```python
from build123d import *

# Parameters (mm, degrees)
SKETCH1_W           = 38
SKETCH1_H           = 26
BOSS_EXTRUDE1_DEPTH = 2
SKETCH4_W           = 29.4
SKETCH4_H           = 21.4
SKETCH4_W_2         = 27.4
SKETCH4_H_2         = 19.4
BOSS_EXTRUDE2_DEPTH = 2
SKETCH5_R           = 3
CUT_EXTRUDE1_DEPTH  = 2


with BuildPart() as part:
    # Sketch1 → Boss-Extrude1 (new body)
    with BuildSketch(Plane.XY):
        Rectangle(SKETCH1_W, SKETCH1_H)
    extrude(amount=BOSS_EXTRUDE1_DEPTH)

    # Sketch4 → Boss-Extrude2 (add)
    with BuildSketch(Plane.XY.offset(2)):
        Rectangle(SKETCH4_W, SKETCH4_H)
        Rectangle(SKETCH4_W_2, SKETCH4_H_2, mode=Mode.SUBTRACT)
    extrude(amount=BOSS_EXTRUDE2_DEPTH)

    # Sketch5 → Cut-Extrude1 (cut)
    with BuildSketch(Plane.XY.offset(2)):
        with Locations((8.600842855, -4.556950786)):
            Circle(SKETCH5_R)
    extrude(amount=-CUT_EXTRUDE1_DEPTH, mode=Mode.SUBTRACT)


solid = part.part
```
Read the model definition and answer for the solid it produces. Units are mm, in the model's axes. A direction names the side the tool comes from. Round coordinates to 2 decimals unless told otherwise and drop trailing zeros. Write each loop counter-clockwise with the first axis right and the second up, starting at its lowest first coordinate (ties: lowest second). Pieces come first, ordered by that corner, then holes. Notation, with made-up numbers: (19.5, -27.5) - (75.5, -27.5) arc R21 cw to (75.5, 0.5) - close; hole circle Ø2 at (72.5, 65.25). An arc over 180 degrees is marked (long way). One line per item, written item: value.
Q1. Straight lines are drawn through the part: line 1 (Y direction, x = 12, z = 2.5); line 2 (X direction, y = -2.5, z = 2.25); line 3 (Z direction, x = -13, y = -12). For each, find the intervals that lie inside material, in ascending order. Write a range as from..to.
The answers:
line 1: y = -10.7..-9.7, 9.7..10.7
line 2: x = -14.7..-13.7, 13.7..14.7
line 3: z = 0..2
Q2. Which of the six approach directions +Z, -Z, +X, -X, +Y, -Y give full straight-line access (tool end or side, diameter ignored) to faces 4 (the flat face through (-14.7, 0, 3)), 5 (the flat face through (0, -10.7, 3)), 6 (the flat face through (0, 9.7, 3)), 7 (the flat face through (0, 10.7, 3)), 8 (the flat face through (14.7, 0, 3))?
The answers:
face 4: +Z, -X, +Y, -Y
face 5: +Z, +X, -X, -Y
face 6: +Z
face 7: +Z, +X, -X, +Y
face 8: +Z, +X, +Y, -Y
Q3. Each of these flat-tipped pins is pushed along its axis until it touches: P1, Ø1.6, axis at x = -4.5, z = 3, coming from the +Y side; P2, Ø0.6, axis at y = -2, z = 3.5, coming from the +X side; P3, Ø13, axis at x = -0.5, y = -2, coming from the +Z side. Where does it stop, or does it pass through?
The answers:
P1: stops at y = 10.7
P2: stops at x = 14.7
P3: stops at z = 2
Q4. Find section B-B (x = 3). Determine the outline of the cut face in (y, z), and give its area (3 significant figures).
The answers:
outline: (-13, 0) - (13, 0) - (13, 2) - (10.7, 2) - (10.7, 4) - (9.7, 4) - (9.7, 2) - (-9.7, 2) - (-9.7, 4) - (-10.7, 4) - (-10.7, 2) - (-13, 2) - close
area: 56.0 mm2
Q5. For a pull along Y with two mould halves and no side action, classify faces 1 (the flat face through (0, 0, 0)), 2 (the flat face through (0, -13, 1)), 3 (the flat face through (13.7, 0, 3)) as pulls with the +Y half, pulls with the -Y half, needs draft (parallel to the pull), parting line crosses it, or undercut.
The answers:
face 1: needs draft
face 2: pulls with the -Y half
face 3: undercut
Q6. Find section C-C (z = 3.2). Determine the outline of the cut face in (x, y), and give its area (3 significant figures).
The answers:
outline: (-14.7, -10.7) - (14.7, -10.7) - (14.7, 10.7) - (-14.7, 10.7) - close; hole (-13.7, -9.7) - (13.7, -9.7) - (13.7, 9.7) - (-13.7, 9.7) - close
area: 97.6 mm2
Q7. Find section A-A (y = 4.25). Determine the outline of the cut face in (x, z).
The answers:
outline: (-19, 0) - (19, 0) - (19, 2) - (14.7, 2) - (14.7, 4) - (13.7, 4) - (13.7, 2) - (-13.7, 2) - (-13.7, 4) - (-14.7, 4) - (-14.7, 2) - (-19, 2) - close
Q8. Find section D-D (x = 7.5). Determine the outline of the cut face in (y, z), and give its area (3 significant figures).
The answers:
outline: (-13, 0) - (-7.35, 0) - (-7.35, 2) - (-9.7, 2) - (-9.7, 4) - (-10.7, 4) - (-10.7, 2) - (-13, 2) - close; (-1.77, 0) - (13, 0) - (13, 2) - (10.7, 2) - (10.7, 4) - (9.7, 4) - (9.7, 2) - (-1.77, 2) - close
area: 44.8 mm2
